Read the model definition and answer for the solid it produces. Units are mm, in the model's axes. A direction names the side the tool comes from. Round coordinates to 2 decimals unless told otherwise and drop trailing zeros. Write each loop counter-clockwise with the first axis right and the second up, starting at its lowest first coordinate (ties: lowest second). Pieces come first, ordered by that corner, then holes.
from build123d import *

# Parameters (mm, degrees)
BOSS_EXTRUDE1_DEPTH = 3
FILLET1_R           = 1.2
FILLET2_R           = 5
FILLET3_R           = 10
FILLET4_R           = 2.5


with BuildPart() as part:
    # Sketch1 → Boss-Extrude1 (new body)
    with BuildSketch(Plane(origin=(0, 0, 0), x_dir=(1, 0, 0), z_dir=(0, 1, 0))):
        with BuildLine():
            Line((-4.5, 0), (4.5, 0))
            Line((4.5, 0), (4.5, -5.46))
            Line((4.5, -5.46), (9.2, -5.46))
            Line((9.2, -5.46), (9.2, -0.91))
            ThreePointArc((9.2, -0.91), (10.9, 0.79), (12.6, -0.91))
            Line((12.6, -0.91), (12.6, -5.46))
            Line((12.6, -5.46), (15.84, -5.46))
            Line((15.84, -5.46), (15.84, 2.73))
            Line((15.84, 2.73), (20.705, 10.95))
            Line((20.705, 10.95), (19.91, 17.44))
            Line((19.91, 17.44), (16.145, 18.62))
            Line((16.145, 18.62), (0, 13.56))
            Line((0, 13.56), (-16.145, 18.62))
            Line((-16.145, 18.62), (-19.91, 17.44))
            Line((-19.91, 17.44), (-20.705, 10.95))
            Line((-20.705, 10.95), (-15.84, 2.73))
            Line((-15.84, 2.73), (-15.84, -5.46))
            Line((-15.84, -5.46), (-12.6, -5.46))
            Line((-12.6, -5.46), (-12.6, -0.91))
            ThreePointArc((-12.6, -0.91), (-10.9, 0.79), (-9.2, -0.91))
            Line((-9.2, -0.91), (-9.2, -5.46))
            Line((-9.2, -5.46), (-4.5, -5.46))
            Line((-4.5, -5.46), (-4.5, 0))
        make_face()
    extrude(amount=BOSS_EXTRUDE1_DEPTH)

    # Fillet1
    fillet1_edges = [part.edges().sort_by_distance(p)[0] for p in [
        (4.5, 1.5, 0),
        (-4.5, 1.5, 0),
        (-9.2, 1.5, 5.46),
        (-15.84, 1.5, 5.46),
        (15.84, 1.5, 5.46),
        (9.2, 1.5, 5.46),
    ]]
    fillet(fillet1_edges, radius=FILLET1_R)

    # Fillet2
    fillet2_edges = [part.edges().sort_by_distance(p)[0] for p in [
        (-16.145, 1.5, -18.62),
        (16.145, 1.5, -18.62),
    ]]
    fillet(fillet2_edges, radius=FILLET2_R)

    # Fillet3
    fillet3_edges = [part.edges().sort_by_distance(p)[0] for p in [
        (-15.84, 1.5, -2.73),
        (-20.705, 1.5, -10.95),
        (0, 1.5, -13.56),
        (20.705, 1.5, -10.95),
        (15.84, 1.5, -2.73),
    ]]
    fillet(fillet3_edges, radius=FILLET3_R)

    # Fillet4
    fillet4_edges = [part.edges().sort_by_distance(p)[0] for p in [
        (-19.91, 1.5, -17.44),
        (19.91, 1.5, -17.44),
    ]]
    fillet(fillet4_edges, radius=FILLET4_R)


solid = part.part
Q1. Section D-D (z = -1.25) is taken. Determine the outline of the cut face in (x, y).
Verdict:
outline: (-15.92, 0) - (15.92, 0) - (15.92, 3) - (-15.92, 3) - close
Q2. Which of the six approach directions +Z, -Z, +X, -X, +Y, -Y give full straight-line access (tool end or side, diameter ignored) to faces 1 (the flat face through (4.5, 1, 3)), 2 (the cylindrical face through (-0.04, 1.52, -14.04))?
Verdict:
face 1: +Z, +Y, -Y
face 2: -Z, +Y, -Y
Q3. Flat-ended cylindrical pins translate along their axes: pin 1 Ø1.5 at (y, z) = (1, 2.5) entering from -X; pin 2 Ø0.9 at (y, z) = (1.5, 3) entering from +X. Find the tip coordinate at first contact, or state that the pin passes through.
Verdict:
pin 1: stops at x = -15.84
pin 2: stops at x = 15.84
Q4. Straight lines are drawn through the part: probe 1 along Z at (x, y) = (3, 0.65); probe 2 along X at (y, z) = (2.5, -1); probe 3 along Z at (x, y) = (8.5, 1.5). For each, find the intervals that lie inside material, in ascending order.
Verdict:
probe 1: z = -14.5 to 0
probe 2: x = -15.89 to 15.89
probe 3: z = -16.22 to 5.35
Q5. Determine the mould class of faces 3 (the flat face through (0, 1, 0)), 4 (the cylindrical face through (-16.17, 1.52, -18.38)), 5 (the flat face through (15.84, 1, 2)), 6 (the cylindrical face through (-15.498, 1.521, 5.099)) for opening direction X: pulls with the +X half, pulls with the -X half, needs draft (parallel to the pull), parting line crosses it, or undercut.
Verdict:
face 3: undercut
face 4: undercut
face 5: pulls with the +X half
face 6: pulls with the -X half
Q6. Section C-C (x = -10.9) is taken. Determine the outline of the cut face in (y, z), then the cut area to 3 significant figures.
Verdict:
outline: (0, -16.98) - (3, -16.98) - (3, -0.79) - (0, -0.79) - close
area: 48.6 mm2
Q7. Section A-A (z = 2) is taken. Determine the outline of the cut face in (x, y), then the cut area to 3 significant figures.
Verdict:
outline: (-15.84, 0) - (-12.6, 0) - (-12.6, 3) - (-15.84, 3) - close; (-9.2, 0) - (-4.5, 0) - (-4.5, 3) - (-9.2, 3) - close; (4.5, 0) - (9.2, 0) - (9.2, 3) - (4.5, 3) - close; (12.6, 0) - (15.84, 0) - (15.84, 3) - (12.6, 3) - close
area: 47.6 mm2
Q8. Section B-B (z = -17) is taken. Determine the outline of the cut face in (x, y).
Verdict:
outline: (-19.65, 0) - (-10.98, 0) - (-10.98, 3) - (-19.65, 3) - close; (10.98, 0) - (19.65, 0) - (19.65, 3) - (10.98, 3) - close
